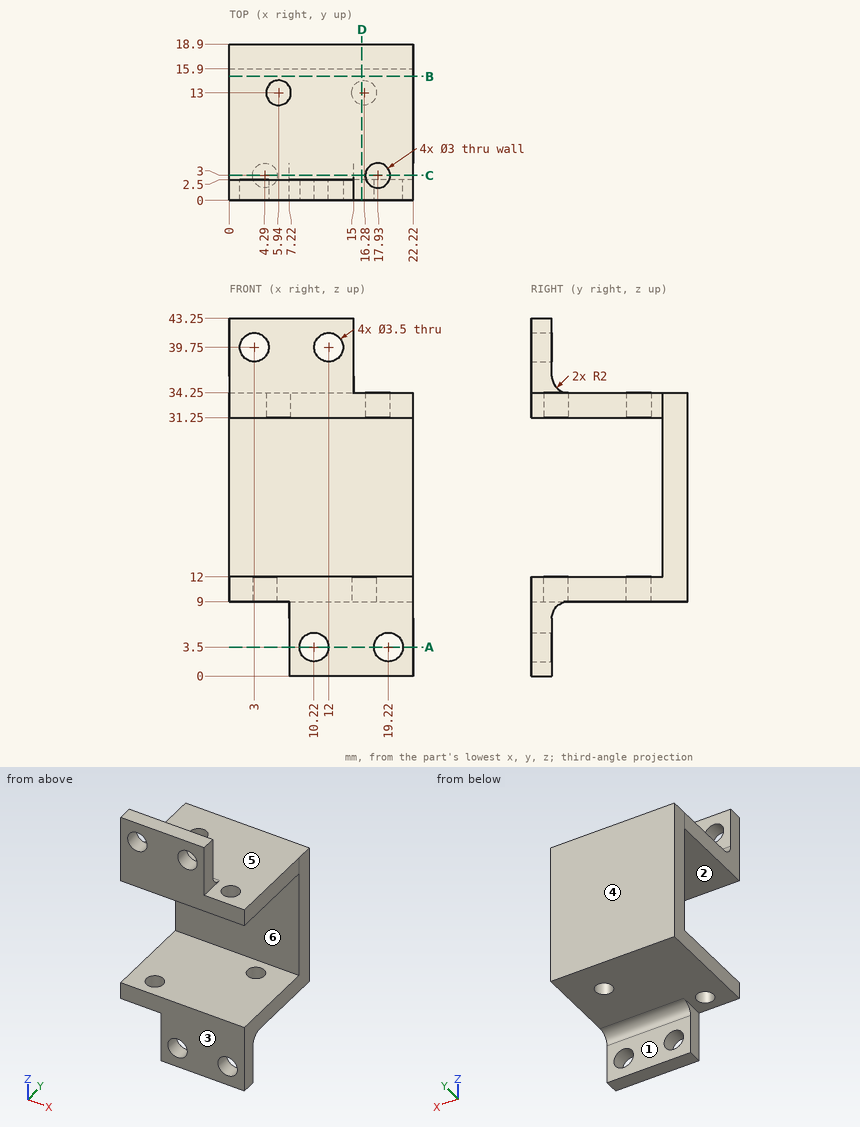
Drawing for the job (mm, zero at the part's lowest x, y, z). A direction names the side the tool comes from. Round coordinates to 2 decimals unless told otherwise and drop trailing zeros. Write each loop counter-clockwise with the first axis right and the second up, starting at its lowest first coordinate (ties: lowest second). Pieces come first, ordered by that corner, then holes. Notation, with made-up numbers: M 34.5,-36.5 L 74.5,-36.5 A25 cw 74.5,1.5 Z; hole C 81.25,67 d2. An arc over 180 degrees is marked long. Answer as a JSON object with one key per item and string values. Group by question number.
(1) Cut at D-D (x = 16). Give the cut face in (y, z).
(2) Mould opens along Z. For the marked faces 4, 5 and 6 say: pulls with the +Z half, pulls with the -Z half, needs draft (parallel to the pull), parting line crosses it, or undercut.
(3) Cut at A-A (z = 3.5). Give the cut face in (x, y).
(4) Flat gauge pins, fed straight in: pin 1 (8 mm diameter, centred on x = 6, z = 27, fed in from -Y); pin 2 (3.5 mm diameter, centred on y = 2.5, z = 6.5, fed in from -X); pin 3 (1 mm diameter, centred on x = 16, y = 13, fed in from -Z). Where does each tip first touch, or does it go through?
(5) Drill centre lines: L1, parallel to Z at x = 3, y = 0.65; L2, parallel to Z at x = 5.5, y = 11.25; L3, parallel to Y at x = 17.5, z = 24.5. Where is each one in solid material? Low to high.
(6) Which spindle directions (+Z, -Z, +X, -X, +Y, -Y) get a long thin tool onto all of the face, cutting with end or side? Do the marked faces 1, 2 and 3. Say none if no direction does.
(7) Cut at C-C (y = 3). Give the cut face in (x, z).
(8) Cut at B-B (y = 15). Give the cut face in (x, z), and give its area (3 significant figures).
Responses:
{
 "1": {"outline": "M 0,0 L 2.5,0 L 2.5,7 A2 cw 4.5,9 L 11.53,9 L 11.53,12 L 0,12 Z; M 0,31.25 L 15.9,31.25 L 15.9,12 L 14.47,12 L 14.47,9 L 18.9,9 L 18.9,34.25 L 0,34.25 Z"},
 "2": {"face 4": "needs draft", "face 5": "pulls with the +Z half", "face 6": "undercut"},
 "3": {"outline": "M 7.22,0 L 8.47,0 L 8.47,2.5 L 7.22,2.5 Z; M 11.97,0 L 17.47,0 L 17.47,2.5 L 11.97,2.5 Z; M 20.97,0 L 22.22,0 L 22.22,2.5 L 20.97,2.5 Z"},
 "4": {"pin 1": "stops at y = 15.9", "pin 2": "stops at x = 7.22", "pin 3": "stops at z = 31.25"},
 "5": {"L1": "z = 9 to 12, 31.25 to 38, 41.5 to 43.25", "L2": "z = 9 to 12, 31.25 to 34.25", "L3": "y = 15.9 to 18.9"},
 "6": {"face 1": "-Z, +X, -X, +Y", "face 2": "+X, -X, -Y", "face 3": "+Z, -Z, +X, -X, -Y"},
 "7": {"outline": "M 0,9 L 2.79,9 L 2.79,12 L 0,12 Z; M 0,31.25 L 16.43,31.25 L 16.43,34.25 L 15,34.25 L 15,34.93 L 0,34.93 Z; M 5.79,9 L 7.22,9 L 7.22,8.32 L 22.22,8.32 L 22.22,12 L 5.79,12 Z; M 19.43,31.25 L 22.22,31.25 L 22.22,34.25 L 19.43,34.25 Z"},
 "8": {"outline": "M 0,9 L 22.22,9 L 22.22,12 L 0,12 Z; M 0,31.25 L 22.22,31.25 L 22.22,34.25 L 0,34.25 Z", "area": "133 mm2"}
}
